Could you check a few things on this drawing? It's one solid part, dimensions in mm from its lowest x, y, z. Round coordinates to 2 decimals unless told otherwise and drop trailing zeros. Loops run counter-clockwise (first coordinate to the right, second up) from the corner with the lowest first, then second, coordinate; pieces in that order, holes last. Notation, with made-up numbers: M 78.25,44.25 L 98.25,44.25 A13 ccw 98.25,56.25 Z; hole C 58.25,61 d11. An arc over 180 degrees is marked long. Write item = value, one per line. Start each with the question number.
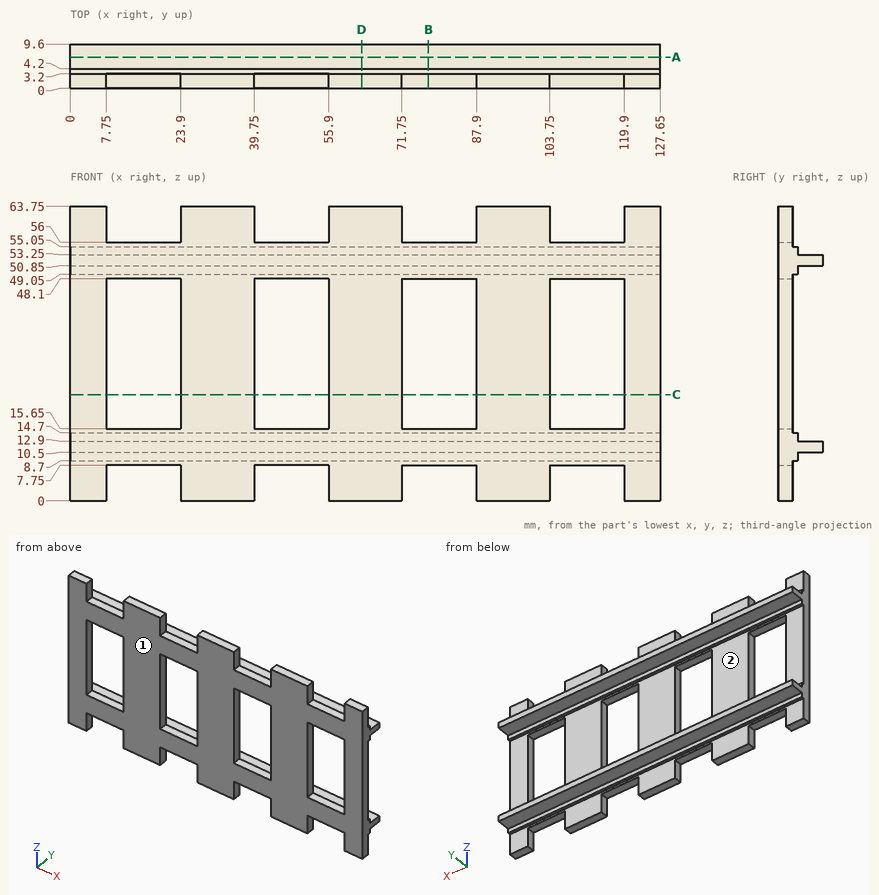
Item 1: I want a section at D-D, the plane x = 63. List the corners of the cut face in (y, z) for me.
Item 2: Please list where these lines run through material, in increasing order: line 1 (X direction, y = 1, z = 31.5); line 2 (Z direction, x = 109.5, y = 9); line 3 (Z direction, x = 115, y = 3). Write a range as [from, to].
Item 3: I want a section at B-B, the plane x = 77.5. List the corners of the cut face in (y, z) for me.
Item 4: We'd pull the mould along Z, two halves only. Please class the marked faces 1 and 2: released by +Z, released by -Z, zero draft, split by the parting line, or undercut.
Item 5: Will these pins go through, and if not, where does the flat tip stop? pin 1 Ø1 at (x, y) = (45.5, 1) entering from -Z; pin 2 Ø0.5 at (x, z) = (55.5, 13.5) entering from +Y; pin 3 Ø1 at (x, y) = (78, 2) entering from +Z.
Item 6: I want a section at A-A, the plane y = 6.75. List the corners of the cut face in (x, z) for me.
Item 7: I want a section at C-C, the plane z = 23. List the corners of the cut face in (x, y) for me, then the cut area to 3 significant figures.
Worked out:
q1.outline = M 0,0 L 3.2,0 L 3.2,8.7 L 4.2,8.7 L 4.2,10.5 L 9.6,10.5 L 9.6,12.9 L 4.2,12.9 L 4.2,14.7 L 3.2,14.7 L 3.2,49.05 L 4.2,49.05 L 4.2,50.85 L 9.6,50.85 L 9.6,53.25 L 4.2,53.25 L 4.2,55.05 L 3.2,55.05 L 3.2,63.75 L 0,63.75 Z
q2.line_1 = [0, 7.75], [23.9, 39.75], [55.9, 71.75], [87.9, 103.75], [119.9, 127.65]
q2.line_2 = [10.5, 12.9], [50.85, 53.25]
q2.line_3 = [7.75, 15.65], [48.1, 56]
q3.outline = M 0,7.75 L 3.2,7.75 L 3.2,8.7 L 4.2,8.7 L 4.2,10.5 L 9.6,10.5 L 9.6,12.9 L 4.2,12.9 L 4.2,14.7 L 3.2,14.7 L 3.2,15.65 L 0,15.65 Z; M 0,48.1 L 3.2,48.1 L 3.2,49.05 L 4.2,49.05 L 4.2,50.85 L 9.6,50.85 L 9.6,53.25 L 4.2,53.25 L 4.2,55.05 L 3.2,55.05 L 3.2,56 L 0,56 Z
q4.face_1 = zero draft
q4.face_2 = undercut
q5.pin_1 = 7.75
q5.pin_2 = 4.2
q5.pin_3 = 56
q6.outline = M 0,10.5 L 127.65,10.5 L 127.65,12.9 L 0,12.9 Z; M 0,50.85 L 127.65,50.85 L 127.65,53.25 L 0,53.25 Z
q7.outline = M 0,0 L 7.75,0 L 7.75,3.2 L 0,3.2 Z; M 23.9,0 L 39.75,0 L 39.75,3.2 L 23.9,3.2 Z; M 55.9,0 L 71.75,0 L 71.75,3.2 L 55.9,3.2 Z; M 87.9,0 L 103.75,0 L 103.75,3.2 L 87.9,3.2 Z; M 119.9,0 L 127.65,0 L 127.65,3.2 L 119.9,3.2 Z
q7.area = 202 mm2
